Work out the finished part from the listing and answer in its coordinate system (mm). Face numbers are marked on the shaded views. A direction names the side the tool comes from. Give positions to 0.01 mm unless a question says otherwise; leave off trailing zeros. Write each loop counter-clockwise with the first axis right and the second up, starting at its lowest first coordinate (ties: lowest second). Pieces come first, ordered by that corner, then holes. Notation, with made-up numbers: (36.5, 67) -> (58.5, 67) arc R20 cw to (58.5, 105) -> close; hole circle Ø1 at (-17.75, -32). An arc over 180 degrees is marked (long way). Use a Markdown table: item, result. Add a question column.
Q1. Each of these flat-tipped pins is pushed along its axis until it touches: pin 1 Ø2 at (y, z) = (0, 2.5) entering from +X; pin 2 Ø4.5 at (y, z) = (-1.5, 0.5) entering from +X; pin 3 Ø3 at (x, y) = (2.5, -2) entering from -Z. Where does it stop, or does it pass through?
Q2. For the marked faces 5 and 6, determine the directions among +Z, -Z, +X, -X, +Y, -Y from which every point of the face is accessible in a straight line to the end or side of a thin tool.
Q3. For a pull along X with two mould halves and no side action, classify the marked faces 1, 2, 3 and 4 as pulls with the +X half, pulls with the -X half, needs draft (parallel to the pull), parting line crosses it, or undercut.
Q4. Consider line 1 (X direction, y = 2.25, z = -4.25); line 2 (X direction, y = -1.75, z = -3.75); line 3 (Y direction, x = 3.5, z = 1.5). Determine where each line is inside the solid, lowest interval first.
Q5. Section A-A, the plane x = -2.5 is taken. Give the vertices of the cut face in (y, z) (3 decimals).
from build123d import *

# Parameters (mm, degrees)
F0_R     = 5
F1_DEPTH = 4.4
F2_R     = 3.175
F3_DEPTH = 1.6
F5_R     = 2.95
F6_DEPTH = 0.6
F8_R     = 4.275
F9_DEPTH = 2.95


with BuildPart() as f1:
    # F0 (on Right) → F1 (new body)
    with BuildSketch(Plane.YZ):
        Circle(F0_R)
    extrude(amount=F1_DEPTH)

    # F2 (on Right) → F3 (join)
    with BuildSketch(Plane.YZ):
        Circle(F2_R)
    extrude(amount=-F3_DEPTH)

    # F5 (on offset) → F6 (join)
    with BuildSketch(Plane.YZ.offset(-1.6)):
        Circle(F5_R)
    extrude(amount=-F6_DEPTH)

    # F8 (on offset) → F9 (join)
    with BuildSketch(Plane.YZ.offset(-2.2)):
        Circle(F8_R)
    extrude(amount=-F9_DEPTH)

    # F10 (on Front) → F11 (revolve, cut)
    with BuildSketch(Plane.XZ):
        with BuildLine():
            Line((4.4, 0), (4.4, 4.5))
            ThreePointArc((4.4, 4.5), (2.77944, 2.504496), (2.2, 0))
            Line((2.2, 0), (4.4, 0))
        make_face()
    revolve(axis=Axis((3.3, 0, 0), (-1, 0, 0)), mode=Mode.SUBTRACT)


solid = f1.part
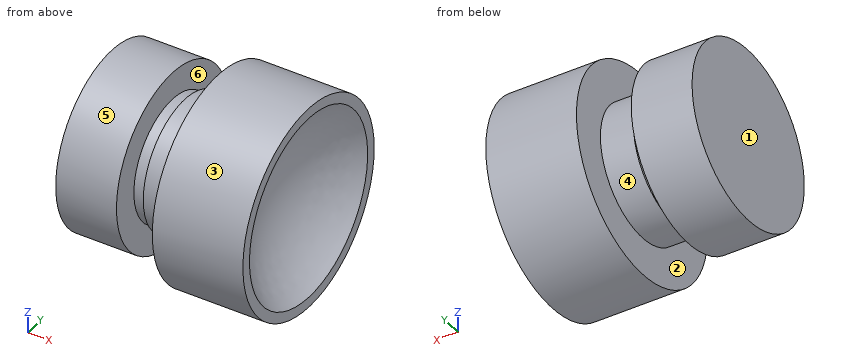
Result set:
| question | item | result |
|---|---|---|
| 1 | pin 1 | stops at x = 3.4 |
| 1 | pin 2 | stops at x = 3.68 |
| 1 | pin 3 | stops at z = -4.97 |
| 2 | face 5 | -X |
| 2 | face 6 | none |
| 3 | face 1 | pulls with the -X half |
| 3 | face 2 | undercut |
| 3 | face 3 | needs draft |
| 3 | face 4 | undercut |
| 4 | line 1 | x = 0 to 4.4 |
| 4 | line 2 | x = -5.15 to -2.2, 0 to 3.98 |
| 4 | line 3 | y = -4.77 to -3.3, 3.3 to 4.77 |
| 5 | outline | circle Ø8.55 at (0, 0) |
